The listing builds one solid part. Answer for the finished solid, in the listing's coordinates (mm). A direction names the side the tool comes from. Give positions to 0.01 mm unless a question says otherwise; leave off trailing zeros. Write each loop counter-clockwise with the first axis right and the second up, starting at its lowest first coordinate (ties: lowest second). Pieces come first, ordered by that corner, then holes. Notation, with made-up numbers: M 71,-27 L 86,-27 A13 ccw 86,-7 Z; hole C 89.5,39 d8. An arc over 180 degrees is marked long. Answer as a JSON object with one key per item and string values.
```python
from build123d import *

# Parameters (mm, degrees)
F0_R     = 25.4
F1_DEPTH = 12.7
F2_R     = 6.35
F3_DEPTH = 50.8
F4_R     = 3.175
F5_DEPTH = 12.7


with BuildPart() as f1:
    # F0 (on Front) → F1 (new body)
    with BuildSketch(Plane.XZ):
        Circle(F0_R)
    extrude(amount=F1_DEPTH)

    # F2 (on face) → F3 (cut)
    with BuildSketch(Plane.XZ.offset(12.7)):
        Circle(F2_R)
    extrude(amount=-F3_DEPTH, mode=Mode.SUBTRACT)

    # F4 (on face) → F5 (join)
    with BuildSketch(Plane.XZ.offset(12.7)):
        with Locations((0, 18.11257)):
            Circle(F4_R)
        with Locations((-15.685946, 9.056285)):
            Circle(F4_R)
        with Locations((-15.685946, -9.056285)):
            Circle(F4_R)
        with Locations((0, -18.11257)):
            Circle(F4_R)
        with Locations((15.685946, -9.056285)):
            Circle(F4_R)
        with Locations((15.685946, 9.056285)):
            Circle(F4_R)
    extrude(amount=F5_DEPTH)


solid = f1.part
```
1. Flat-ended cylindrical pins translate along their axes: pin 1 (2 mm diameter, centred on y = -8, z = -14.5, fed in from -X); pin 2 (2 mm diameter, centred on x = -8, y = -3, fed in from +Z); pin 3 (1.5 mm diameter, centred on y = -15, z = -12.5, fed in from -X); pin 4 (1.5 mm diameter, centred on x = 5.5, y = -14.5, fed in from -Z). Find the tip coordinate at first contact, or state that the pin passes through.
Verdict:
{"pin 1": "stops at x = -21.52", "pin 2": "stops at z = 24.42", "pin 3": "stops at x = -17.37", "pin 4": "passes through"}
2. Consider line 1 along Z through (x, y) = (0, -4); line 2 along Y through (x, z) = (-22, 3); line 3 along Z through (x, y) = (-18, -17). Determine where each line is inside the solid, lowest interval first.
Verdict:
{"line 1": "z = -25.4 to -6.35, 6.35 to 25.4", "line 2": "y = -12.7 to 0", "line 3": "z = -11.23 to -6.88, 6.88 to 11.23"}
3. A cutting plane is placed at D-D, the plane x = -17. Give the vertices of the cut face in (y, z), plus the area to 3 significant figures.
Verdict:
{"outline": "M -25.4,-11.95 L -12.7,-11.95 L -12.7,-18.87 L 0,-18.87 L 0,18.87 L -12.7,18.87 L -12.7,11.95 L -25.4,11.95 L -25.4,6.17 L -12.7,6.17 L -12.7,-6.17 L -25.4,-6.17 Z", "area": "626 mm2"}
4. The mould has two halves that part along X. Classify faces 1 (the cylindrical face through (-0.413, -18.961, -14.965)), 2 (the flat face through (16, -25.4, -9)), 3 (the cylindrical face through (18.714, -18.961, -8.103)): released by +X, released by -X, zero draft, split by the parting line, or undercut.
Verdict:
{"face 1": "split by the parting line", "face 2": "zero draft", "face 3": "undercut"}
5. A cutting plane is placed at C-C, the plane y = -18.25. Give the vertices of the cut face in (x, z) (3 decimals), plus the area to 3 significant figures.
Verdict:
{"outline": "C -15.686,-9.056 d6.35; C -15.686,9.056 d6.35; C 0,-18.113 d6.35; C 0,18.113 d6.35; C 15.686,-9.056 d6.35; C 15.686,9.056 d6.35", "area": "190 mm2"}
6. For faces 4 (the cylindrical face through (-0.41, -18.96, 21.26)), 5 (the flat face through (0, -25.4, 18)), determine the directions among +Z, -Z, +X, -X, +Y, -Y from which every point of the face is accessible in a straight line to the end or side of a thin tool.
Verdict:
{"face 4": "-Y", "face 5": "+Z, -Z, +X, -X, -Y"}
7. A cutting plane is placed at B-B, the plane z = 1.5. Give the vertices of the cut face in (x, y), plus the area to 3 significant figures.
Verdict:
{"outline": "M -25.36,-12.7 L -6.17,-12.7 L -6.17,0 L -25.36,0 Z; M 6.17,-12.7 L 25.36,-12.7 L 25.36,0 L 6.17,0 Z", "area": "487 mm2"}
8. A cutting plane is placed at A-A, the plane x = 0. Give the vertices of the cut face in (y, z).
Verdict:
{"outline": "M -25.4,-21.29 L -12.7,-21.29 L -12.7,-25.4 L 0,-25.4 L 0,-6.35 L -12.7,-6.35 L -12.7,-14.94 L -25.4,-14.94 Z; M -25.4,14.94 L -12.7,14.94 L -12.7,6.35 L 0,6.35 L 0,25.4 L -12.7,25.4 L -12.7,21.29 L -25.4,21.29 Z"}
